The listing builds one solid part. Answer for the finished solid, in the listing's coordinates (mm). Face numbers are marked on the shaded views. Coordinates: 2 decimals unless noted, no trailing zeros. Order: outer loops, then holes, each group sorted by start corner. A loop starts at its lowest first (then second) coordinate and runs counter-clockwise, first axis right, second up. Notation, with made-up numbers: (48, 6) - (93, 6) arc R33 cw to (93, 40) - close; hole circle Ø9 at (60, 31). An arc over 180 degrees is marked (long way). Use one line per item in the form item = value. Start each with the question number.
Item 1: Section A-A, the plane z = 0 is taken. Write down the section's boundary in (x, y).
Item 2: Each of these flat-tipped pins is pushed along its axis until it touches: pin 1 Ø3.5 at (x, z) = (1.21, 0) entering from +Y; pin 2 Ø1.5 at (y, z) = (-5.5, 1) entering from +X; pin 3 Ø2 at (y, z) = (-5.5, 5.5) entering from +X; pin 4 Ø4 at (x, y) = (7, -4.5) entering from -Z. Where does it stop, or does it pass through?
Item 3: Consider line 1 along Z through (x, y) = (1.25, -1.5); line 2 along Y through (x, z) = (-2, 5.5); line 3 along Z through (x, y) = (0, -3.5). Determine where each line is inside the solid, lowest interval first. Write a range as [from, to].
Item 4: The mould has two halves that part along Z. Classify the marked faces 1, 2 and 3: released by +Z, released by -Z, zero draft, split by the parting line, or undercut.
Item 5: Section B-B, the plane y = -2.75 is taken. Write down the section's boundary in (x, z), and give its area (3 significant figures).
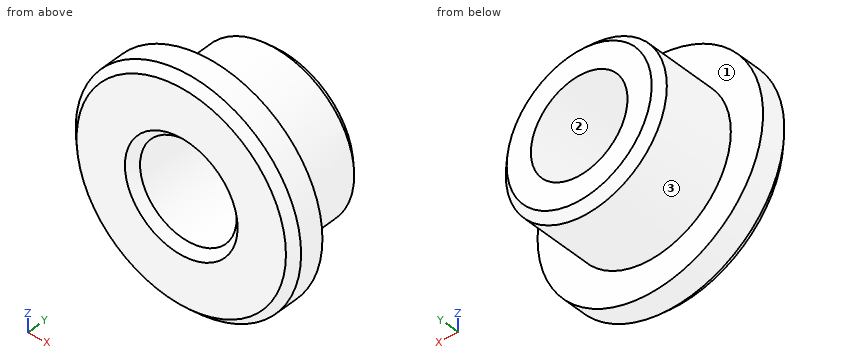
from build123d import *

# Parameters (mm, degrees)
F0_R     = 5
F0_R_2   = 3
F1_DEPTH = 5
F2_R     = 6.9999998716
F2_R_2   = 5
F2_R_3   = 3
F3_DEPTH = 2
F4_SIZE  = 0.5
F5_SIZE  = 0.5
F6_SIZE  = 0.5


with BuildPart() as f1:
    # F0 (on Front) → F1 (new body)
    with BuildSketch(Plane.XZ):
        with Locations((1.2148135622, 0)):
            Circle(F0_R)
        with Locations((1.2148135622, 0)):
            Circle(F0_R_2, mode=Mode.SUBTRACT)
    extrude(amount=F1_DEPTH)

    # F2 (on face) → F3 (join)
    with BuildSketch(Plane.XZ.offset(5)):
        with Locations((1.2148135622, 0)):
            Circle(F2_R)
        with Locations((1.2148135622, 0)):
            Circle(F2_R_2, mode=Mode.SUBTRACT)
        with Locations((1.2148135622, 0)):
            Circle(F2_R_2)
        with Locations((1.2148135622, 0)):
            Circle(F2_R_3, mode=Mode.SUBTRACT)
    extrude(amount=F3_DEPTH)

    # F4
    f4_edges = [f1.edges().sort_by_distance(p)[0] for p in [
        (-1.785186, -7, 0),
    ]]
    chamfer(f4_edges, length=F4_SIZE)

    # F5
    f5_edges = [f1.edges().sort_by_distance(p)[0] for p in [
        (-5.785186, -7, 0),
    ]]
    chamfer(f5_edges, length=F5_SIZE)

    # F6
    f6_edges = [f1.edges().sort_by_distance(p)[0] for p in [
        (-3.785186, 0, 0),
    ]]
    chamfer(f6_edges, length=F6_SIZE)


solid = f1.part
Response:
q1.outline = (-5.79, -6.5) - (-5.29, -7) - (-2.29, -7) - (-1.79, -6.5) - (-1.79, 0) - (-3.29, 0) - (-3.79, -0.5) - (-3.79, -5) - (-5.79, -5) - close; (4.21, -6.5) - (4.71, -7) - (7.71, -7) - (8.21, -6.5) - (8.21, -5) - (6.21, -5) - (6.21, -0.5) - (5.71, 0) - (4.21, 0) - close
q2.pin_1 = through
q2.pin_2 = 8.21
q2.pin_3 = 6.58
q2.pin_4 = -5.85
q3.line_1 = [-5, -3], [3, 5]
q3.line_2 = [-7, -5]
q3.line_3 = [-4.85, -2.74], [2.74, 4.85]
q4.face_1 = zero draft
q4.face_2 = undercut
q4.face_3 = split by the parting line
q5.outline = circle Ø10 at (1.21, 0); hole circle Ø6 at (1.21, 0)
q5.area = 50.3 mm2
